Autodesk Inventor part; units mm, degrees
ref_plane "YZ Plane" through (0, 0, 0) normal (1, 0, 0) x (0, 1, 0)
ref_plane "XZ Plane" through (0, 0, 0) normal (0, 1, 0) x (-1, 0, 0)
ref_plane "XY Plane" through (0, 0, 0) normal (0, 0, 1) x (1, 0, 0)
sketch "Sketch1" plane through (0, 0, 0) normal (0, 1, 0) x (-1, 0, 0)
  line L0 (0, 0) -> (48.26, 0)
  line L1 (48.26, 0) -> (48.26, -20.32)
  line L2 (48.26, -20.32) -> (0, -20.32)
  line L3 (0, -20.32) -> (0, 0)
  line L4 (33.02, -2.6035) -> (13.97, -2.6035)
  line L5 (13.97, -2.6035) -> (13.97, -17.8435)
  line L6 (13.97, -17.8435) -> (33.02, -17.8435)
  line L7 (33.02, -17.8435) -> (33.02, -2.6035)
  dimension "d0" = 48.26
  dimension "d1" = 20.32
  dimension "d2" = 19.05
  dimension "d3" = 15.24
  dimension "d4" = 15.24
  dimension "d5" = 2.6035
extrude "Extrusion1" add sketch "Sketch1" along normal blind 1.905
sketch "Sketch2" plane through (-48.26, 0, 0) normal (0, 0, 1) x (1, 0, 0)
  line L0 (48.26, 0) -> (0, 0)
  line L1 (48.26, 0) -> (48.26, 1.905)
  line L2 (0, 1.905) -> (48.26, 1.905)
  line L3 (0, 0) -> (0, 1.905)
  circle A0 centre (3.175, 3.937) radius 1.8415
  circle A1 centre (45.085, 3.937) radius 1.8415
  circle A2 centre (3.175, 3.937) radius 3.175
  circle A3 centre (45.085, 3.937) radius 3.175
  line L4 (0, 1.905) -> (48.26, 1.905)
  line L5 (0, 0) -> (0, 1.905)
  line L6 (0, 3.937) -> (0, 1.905)
  line L7 (6.35, 3.937) -> (6.35, 1.905)
  line L8 (48.26, 1.905) -> (0, 1.905)
  line L9 (48.26, 3.937) -> (48.26, 1.905)
  line L10 (41.91, 3.937) -> (41.91, 1.905)
  dimension "d8" = 3.683
  dimension "d9" = 41.91
  dimension "d10" = 6.35
  dimension "d28" = 2.032
extrude "Extrusion2" add sketch "Sketch2" against normal blind 1.905
sketch "Sketch3" plane through (0, 0, -20.32) normal (0, 0, -1) x (-1, 0, 0)
  circle A0 centre (3.175, 3.937) radius 1.8415
  arc A1 (6.35, 3.937) -> (0, 3.937) centre (3.175, 3.937) ccw
  line L0 (0, 3.937) -> (0, 1.905)
  line L1 (6.35, 1.905) -> (0, 1.905)
  line L2 (6.35, 1.905) -> (6.35, 3.937)
  circle A2 centre (45.085, 3.937) radius 1.8415
  line L3 (48.26, 1.905) -> (41.91, 1.905)
  line L4 (48.26, 1.905) -> (48.26, 3.937)
  arc A3 (48.26, 3.937) -> (41.91, 3.937) centre (45.085, 3.937) ccw
  line L5 (41.91, 3.937) -> (41.91, 1.905)
  point P0 (0, 0)
extrude "Extrusion3" add sketch "Sketch3" against normal blind 1.905
sketch "Sketch4" plane through (0, 1.905, 0) normal (0, 1, 0) x (1, 0, 0)
  line L0 (-33.02, 2.6035) -> (-33.02, 17.8435) construction
  circle A0 centre (-36.195, 16.5735) radius 1.8415
  circle A1 centre (-36.195, 10.2235) radius 1.8415
  circle A2 centre (-36.195, 3.8735) radius 1.8415
  line L1 (-36.195, 16.5735) -> (-36.195, 10.2235) construction
  line L2 (-36.195, 10.2235) -> (-36.195, 3.8735) construction
  line L3 (-13.97, 2.6035) -> (-33.02, 2.6035) construction
  point P0 (0, 0)
  dimension "d18" = 3.683
  dimension "d19" = 3.175
  dimension "d20" = 6.35
  dimension "d21" = 1.27
extrude "Extrusion4" cut sketch "Sketch4" against normal through all
sketch "Sketch5" plane through (0, 1.905, 0) normal (0, 1, 0) x (1, 0, 0)
  line L0 (-48.26, 18.415) -> (-41.91, 18.415)
  line L1 (-41.91, 1.905) -> (-48.26, 1.905)
  line L2 (0, 1.905) -> (-6.35, 1.905)
  line L3 (-6.35, 18.415) -> (0, 18.415)
  line L4 (-41.91, 18.415) -> (-48.26, 18.415)
  line L5 (-48.26, 18.415) -> (-40.005, 18.415)
  line L6 (-40.005, 18.415) -> (-40.005, 1.905)
  line L7 (-40.005, 1.905) -> (-48.26, 1.905)
  line L8 (-48.26, 1.905) -> (-48.26, 18.415)
  line L9 (0, 1.905) -> (-8.255, 1.905)
  line L10 (-8.255, 1.905) -> (-8.255, 18.415)
  line L11 (-8.255, 18.415) -> (0, 18.415)
  line L12 (0, 18.415) -> (0, 1.905)
  point P0 (0, 0)
  dimension "d24" = 8.255
extrude "Extrusion5" cut sketch "Sketch5" against normal through all
fillet "Fillet1" radius 1.905 4 edges at (-40.005, 0.9525, -18.415) (-40.005, 0.9525, -1.905) (-8.255, 0.9525, -1.905) (-8.255, 0.9525, -18.415)
chamfer "Chamfer1" distance 1.778 angle 45 4 edges at (-48.26, 0, -19.3675) (-48.26, 0, -0.9525) (0, 0, -0.9525) (0, 0, -19.3675)
properties part number "RelayHolder" material "ABS Plastic"
The listing builds one solid part. Answer for the finished solid, in the listing's coordinates (mm). A direction names the side the tool comes from. Coordinates: 2 decimals unless noted, no trailing zeros. Loops run counter-clockwise (first coordinate to the right, second up) from the corner with the lowest first, then second, coordinate; pieces in that order, holes last. Notation, with made-up numbers: (36.5, -21.5) -> (71.5, -21.5) arc R28 ccw to (71.5, 3.5) -> close; hole circle Ø11 at (0, 47). An arc over 180 degrees is marked (long way). Return JSON: item names as keys, results as strings. Group by question number.
(1) A cutting plane is placed at B-B on z = -13.25. Write down the section's boundary in (x, y) (3 decimals).
(2) A cutting plane is placed at C-C on y = 0.5. Count the separate pieces of the cut face and the enclosed holes in it, and give its area (3 significant figures).
(3) Which of the six approach directions +Z, -Z, +X, -X, +Y, -Y give full straight-line access (tool end or side, diameter ignored) to faces 3 (the flat face through (-23, 1, -17.844)), 4 (the flat face through (-44, 2, -18.415)), 5 (the flat face through (-8.255, 1, -10))?
(4) Determine the mould class of faces 1 (the cylindrical face through (-1.474, 3.232, -0.939)), 2 (the cylindrical face through (-7.712, 0.939, -17.842)) for opening direction Z: released by +Z, released by -Z, zero draft, split by the parting line, or undercut.
(5) Find the intervals of material crossed by probe 1 along Z at (x, y) = (-44.5, 6.75) (3 decimals); probe 2 along X at (y, z) = (5.5, -18.5); probe 3 along X at (y, z) = (3.25, -19.5), in increasing order. Write a range as from..to.
(6) A cutting plane is placed at D-D on x = -35. Write down the section's boundary in (y, z) (3 decimals), and give its area (3 significant figures).
(7) Given pin 1 Ø3.5 at (x, z) = (-36.2, -10.22) entering from +Y; pin 2 Ø2 at (y, z) = (1, -8) entering from +X (3 decimals); pin 3 Ø5 at (x, z) = (-42, -4) entering from +Y; pin 4 Ø1 at (x, z) = (-39.5, -16.5) entering from +Y (3 decimals), each flat-ended and moving along its own axis, determine where each tip first touches the part or whether it passes through.
(8) A cutting plane is placed at A-A on x = -24. Write down the section's boundary in (y, z) (1 decimal), and give its area (3 significant figures).
The answers:
{
 "1": {"outline": "(-40.005, 0) -> (-33.02, 0) -> (-33.02, 1.905) -> (-40.005, 1.905) -> close; (-13.97, 0) -> (-8.255, 0) -> (-8.255, 1.905) -> (-13.97, 1.905) -> close"},
 "2": {"separate pieces": "1", "enclosed holes": "4", "area": "379 mm^2"},
 "3": {"face 3": "+Y, -Y", "face 4": "-X, +Y, -Y", "face 5": "+X, +Y, -Y"},
 "4": {"face 1": "zero draft", "face 2": "undercut"},
 "5": {"probe 1": "z = -20.32..-18.415, -1.905..0", "probe 2": "x = -47.85..-46.06, -44.11..-42.32, -5.94..-4.15, -2.2..-0.41", "probe 3": "x = -48.26..-46.79, -43.38..-41.91, -6.35..-4.88, -1.47..0"},
 "6": {"outline": "(0, -20.32) -> (1.905, -20.32) -> (1.905, -17.975) -> (0, -17.975) -> close; (0, -15.172) -> (1.905, -15.172) -> (1.905, -11.625) -> (0, -11.625) -> close; (0, -8.822) -> (1.905, -8.822) -> (1.905, -5.275) -> (0, -5.275) -> close; (0, -2.472) -> (1.905, -2.472) -> (1.905, 0) -> (0, 0) -> close", "area": "22.7 mm^2"},
 "7": {"pin 1": "passes through", "pin 2": "stops at x = -8.255", "pin 3": "stops at y = 6.61", "pin 4": "stops at y = 1.905"},
 "8": {"outline": "(0, -20.3) -> (1.9, -20.3) -> (1.9, -17.8) -> (0, -17.8) -> close; (0, -2.6) -> (1.9, -2.6) -> (1.9, 0) -> (0, 0) -> close", "area": "9.68 mm^2"}
}
